Design review of the part built by this model. Coordinates are the model's own, in mm. Coordinates: 2 decimals unless noted, no trailing zeros. Loops run counter-clockwise (first coordinate to the right, second up) from the corner with the lowest first, then second, coordinate; pieces in that order, holes last. Notation, with made-up numbers: (0.25, 27.25) - (29.25, 27.25) arc R17 cw to (29.25, 40.25) - close; hole circle Ø10 at (-13.5, -35). An arc over 180 degrees is marked (long way). Answer in a Markdown table with one row per item. Add a question column.
(1) We need section D-D, the plane x = 42.4. Write out the cut boundary in (y, z), plus the area to 3 significant figures.
(2) Clearance check with a flat-ended pin moving along its axis: pin 1 (2.5 mm diameter, centred on x = 42.4, y = 40, fed in from -Z). State where the tip first meets the part, or that it passes through.
(3) We need section B-B, the plane z = 1.2. Give the number of separate pieces and of enclosed holes in the cut face, plus the area to 3 significant figures.
(4) The part is to be moulded in two halves that separate along Y. For faces 1 (the face through (23.484, 9.207, 2.415)), 2 (the face through (49.3, 1.43, 2.41)), 3 (the face through (25, 47, 2)), say which applies: released by +Y, released by -Y, zero draft, split by the parting line, or undercut.
(5) We need section C-C, the plane y = 7.45. Write out the cut boundary in (x, z), plus the area to 3 significant figures.
(6) To check wall thickness, follow L1, parallel to Y at x = 25.4, z = 2.7; L2, parallel to Y at x = 8.4, z = 3.2; L3, parallel to X at y = 39.5, z = 3.25. State the ranges of each line that lie inside material, in increasing order. Write a range as [from, to].
(7) We need section A-A, the plane x = 25.4. Write out the cut boundary in (y, z).
from build123d import *

# Parameters (mm, degrees)
CROQUIS1_W              = 50.8
CROQUIS1_H              = 47
SALIENTE_EXTRUIR1_DEPTH = 4.7625
CROQUIS4_R              = 2.6
CORTAR_EXTRUIR2_DEPTH   = 5.7625
REDONDEO1_R             = 5
CROQUIS7_R              = 1.5875
CORTAR_EXTRUIR5_DEPTH   = 10


with BuildPart() as part:
    # Croquis1 → Saliente-Extruir1 (new body)
    with BuildSketch(Plane.XY):
        with Locations((25.4, 23.5)):
            Rectangle(CROQUIS1_W, CROQUIS1_H)
    extrude(amount=SALIENTE_EXTRUIR1_DEPTH)

    # Croquis4 → Cortar-Extruir2 (cut, through all)
    with BuildSketch(Plane.XY.offset(4.7625)):
        with Locations((25.4, 39.55)):
            Circle(CROQUIS4_R)
        with Locations((25.4, 7.45)):
            Circle(CROQUIS4_R)
    extrude(amount=-CORTAR_EXTRUIR2_DEPTH, mode=Mode.SUBTRACT)

    # Redondeo1
    redondeo1_edges = [part.edges().sort_by_distance(p)[0] for p in [
        (0, 47, 2.38125),
        (50.8, 47, 2.38125),
        (50.8, 0, 2.38125),
        (0, 0, 2.38125),
    ]]
    fillet(redondeo1_edges, radius=REDONDEO1_R)

    # Croquis7 → Cortar-Extruir5 (cut)
    with BuildSketch(Plane.XY.offset(4.7625)):
        with Locations((8.4, 40)):
            Circle(CROQUIS7_R)
        with Locations((42.4, 40)):
            Circle(CROQUIS7_R)
    extrude(amount=-CORTAR_EXTRUIR5_DEPTH, mode=Mode.SUBTRACT)


solid = part.part
Responses:
| question | item | result |
|---|---|---|
| 1 | outline | (0, 0) - (38.41, 0) - (38.41, 4.76) - (0, 4.76) - close; (41.59, 0) - (47, 0) - (47, 4.76) - (41.59, 4.76) - close |
| 1 | area | 209 mm2 |
| 2 | pin 1 | passes through |
| 3 | separate pieces | 1 |
| 3 | enclosed holes | 4 |
| 3 | area | 2,310 mm2 |
| 4 | face 1 | undercut |
| 4 | face 2 | released by -Y |
| 4 | face 3 | released by +Y |
| 5 | outline | (0, 0) - (22.8, 0) - (22.8, 4.76) - (0, 4.76) - close; (28, 0) - (50.8, 0) - (50.8, 4.76) - (28, 4.76) - close |
| 5 | area | 217 mm2 |
| 6 | L1 | y = [0, 4.85], [10.05, 36.95], [42.15, 47] |
| 6 | L2 | y = [0, 38.41], [41.59, 47] |
| 6 | L3 | x = [0, 6.89], [9.91, 22.8], [28, 40.89], [43.91, 50.8] |
| 7 | outline | (0, 0) - (4.85, 0) - (4.85, 4.76) - (0, 4.76) - close; (10.05, 0) - (36.95, 0) - (36.95, 4.76) - (10.05, 4.76) - close; (42.15, 0) - (47, 0) - (47, 4.76) - (42.15, 4.76) - close |
